Geometry: final body of the model. Coordinates: model frame, mm. Face numbers are marked on the shaded views. A direction names the side the tool comes from. Round coordinates to 2 decimals unless told otherwise and drop trailing zeros. Write each loop counter-clockwise with the first axis right and the second up, starting at its lowest first coordinate (ties: lowest second). Pieces come first, ordered by that corner, then holes. Notation, with made-up numbers: (86, -25) - (134, -25) arc R15 cw to (134, -8) - close; hole circle Ø8 at (33.5, -30). An arc over 180 degrees is marked (long way). Write each question's results on one line, items separated by ' | '.
from build123d import *

# Parameters (mm, degrees)
F0_W     = 68.8
F0_H     = 9.54
F0_W_2   = 25.4
F0_H_2   = 2.54
F0_R     = 3.3655
F1_DEPTH = 40
F2_W     = 25.4
F2_H     = 9.525
F3_DEPTH = 3.5
F6_DEPTH = 68.8
F8_DEPTH = 7.62


with BuildPart() as f1:
    # F0 (on Front) → F1 (new body)
    with BuildSketch(Plane.XZ):
        with Locations((31.4, 1.27)):
            Rectangle(F0_W, F0_H)
        with Locations((12.7, 1.27)):
            Rectangle(F0_W_2, F0_H_2, mode=Mode.SUBTRACT)
        with Locations((31.4, 1.27)):
            Circle(F0_R, mode=Mode.SUBTRACT)
        with Locations((50.1, 1.27)):
            Rectangle(F0_W_2, F0_H_2, mode=Mode.SUBTRACT)
    extrude(amount=F1_DEPTH)

    # F2 (on face) → F3 (cut, through all)
    with BuildSketch(Plane(origin=(0, 0, -3.5), x_dir=(1, 0, 0), z_dir=(0, 0, -1))):
        with Locations((12.7, 35.2375)):
            Rectangle(F2_W, F2_H)
        with Locations((50.1, 35.2375)):
            Rectangle(F2_W, F2_H)
    extrude(amount=-F3_DEPTH, mode=Mode.SUBTRACT)

    # F5 (on face) → F6 (cut, through all)
    with BuildSketch(Plane.YZ.offset(65.8)):
        with BuildLine():
            Line((-40, -3.5), (-36.412868955, -3.5))
            add(Edge.make_bspline(
                [(-40, 6.04), (-40, 2.5308377617), (-38.3018730084, -0.3928871964), (-36.412868955, -3.5)],
                knots=[0, 0, 0, 0, 10.1921101414, 10.1921101414, 10.1921101414, 10.1921101414], degree=3))
            Line((-40, 6.04), (-40, -3.5))
        make_face()
    extrude(amount=-F6_DEPTH, mode=Mode.SUBTRACT)

    # F7 (on face) → F8 (join)
    with BuildSketch(Plane(origin=(0, 0, 0), x_dir=(-1, 0, 0), z_dir=(0, 1, 0))):
        with BuildLine():
            ThreePointArc((-37.4, 1.905), (-43.6789598779, 0.4788991858), (-50.1, 0))
            Line((-50.1, 0), (-37.4, 0))
            Line((-37.4, 0), (-37.4, 1.905))
        make_face()
        with BuildLine():
            ThreePointArc((-50.1, 0), (-56.5210401221, 0.4788991858), (-62.8, 1.905))
            Line((-62.8, 1.905), (-62.8, 0))
            Line((-62.8, 0), (-50.1, 0))
        make_face()
        with BuildLine():
            Line((-38.8520723687, 2.54), (-61.3479276313, 2.54))
            ThreePointArc((-61.3479276313, 2.54), (-50.1, 1.016), (-38.8520723687, 2.54))
        make_face()
        with BuildLine():
            ThreePointArc((0, 1.905), (-6.2789599942, 0.4788991684), (-12.7000002352, 0))
            Line((-12.7000002352, 0), (0, 0))
            Line((0, 0), (0, 1.905))
        make_face()
        with BuildLine():
            Line((-25.4, 1.905), (-25.4, 0))
            Line((-25.4, 0), (-12.7000002352, 0))
            ThreePointArc((-12.7000002352, 0), (-19.1210402384, 0.4788992032), (-25.4, 1.905))
        make_face()
        with BuildLine():
            ThreePointArc((-23.9479276313, 2.54), (-12.7, 1.016), (-1.4520723687, 2.54))
            Line((-1.4520723687, 2.54), (-23.9479276313, 2.54))
        make_face()
    extrude(amount=-F8_DEPTH)


solid = f1.part
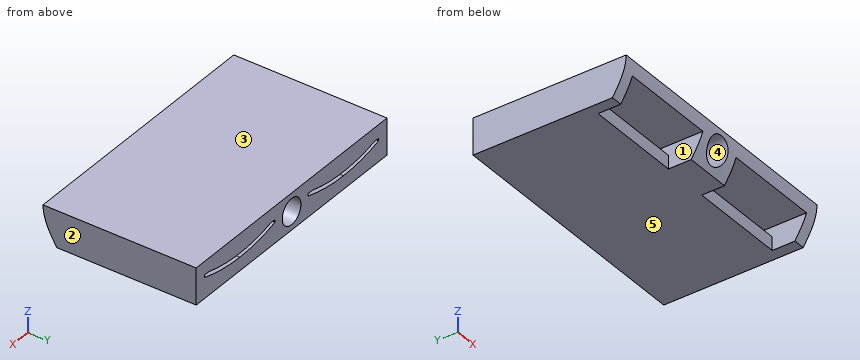
Q1. Mould query, pull axis Z, two halves, no side actions, for the marked faces 3, 4 and 5. Classes: pulls with the +Z half, pulls with the -Z half, needs draft (parallel to the pull), parting line crosses it, or undercut.
Answer block:
face 3: pulls with the +Z half | face 4: undercut | face 5: pulls with the -Z half
Q2. Section query A-A, the plane y = -19.5. Return loops of the section in (x, z).
Answer block:
outline: (-3, -3.5) - (65.8, -3.5) - (65.8, 6.04) - (-3, 6.04) - close; hole (0, 0) - (25.4, 0) - (25.4, 2.54) - (0, 2.54) - close; hole circle Ø6.73 at (31.4, 1.27); hole (37.4, 0) - (62.8, 0) - (62.8, 2.54) - (37.4, 2.54) - close
Q3. Ray query, line 1 along X through (y, z) = (-12.5, 1.27); line 2 along Z through (x, y) = (37.5, -14.5); line 3 along Z through (x, y) = (31.4, -14). Return the intervals inside material, ascending.
Answer block:
line 1: -3 to 0, 25.4 to 28.03, 34.77 to 37.4, 62.8 to 65.8 | line 2: -3.5 to 0, 2.54 to 6.04 | line 3: -3.5 to -2.1, 4.64 to 6.04
Q4. Access query for the marked faces 1 and 2. Directions: +Z, -Z, +X, -X, +Y, -Y. A direction counts if a zero-diameter tool reaches every point of the face in a straight line with its end or side. Return the directions, or none.
Answer block:
face 1: -Y | face 2: +Z, -Z, +X, +Y, -Y
Q5. Pin query (flat end, axial travel): pin 1 (1 mm diameter, centred on x = 6.5, z = -1.5, fed in from -Y) (3 decimals); pin 2 (4 mm diameter, centred on x = 31.4, z = 1.27, fed in from -Y); pin 3 (0.6 mm diameter, centred on x = 46.5, z = 1, fed in from -Y); pin 4 (1.7 mm diameter, centred on x = 9, z = 2, fed in from -Y). Return the tip coordinate at first contact, or that it passes through.
Answer block:
pin 1: y = -30.475 | pin 2: through | pin 3: y = -7.62 | pin 4: y = -39.53
